```python
from build123d import *

# Parameters (mm, degrees)
BOSS_EXTRUDE2_DEPTH = 25
SKETCH4_R           = 4
CUT_EXTRUDE1_DEPTH  = 108.5257706
SKETCH6_R           = 4
CUT_EXTRUDE2_DEPTH  = 78.032036302
CUT_EXTRUDE3_DEPTH  = 78.032036302
SKETCH9_R           = 1.5
CUT_EXTRUDE4_DEPTH  = 78.032036302
SKETCH10_R          = 1.5
CUT_EXTRUDE5_DEPTH  = 108.5257706


with BuildPart() as part:
    # Sketch3 → Boss-Extrude2 (new body)
    with BuildSketch(Plane.XY):
        Polygon((-79.925523148, 45.386502584), (-27.042967192, 45.386502584), (-24.925523148, 45.386502584), (-24.925523148, -19.613497416), (-26.925523148, -19.613497416), (-26.925523148, 43.389953837), (-79.925523148, 43.389953837), (-79.925523148, -19.613497416), (-81.925523148, -19.613497416), (-81.925523148, 45.386502584), align=None)
    extrude(amount=BOSS_EXTRUDE2_DEPTH)

    # Sketch4 → Cut-Extrude1 (cut, through all)
    with BuildSketch(Plane(origin=(0, 45.386502584, 0), x_dir=(1, 0, 0), z_dir=(0, 1, 0))):
        with Locations(Location((-53.425523148, -12.5, 0), (0, 0, 270))):
            Circle(SKETCH4_R)
    extrude(amount=-CUT_EXTRUDE1_DEPTH, mode=Mode.SUBTRACT)

    # Sketch6 → Cut-Extrude2 (cut, through all)
    with BuildSketch(Plane.ZY.offset(81.925523148)):
        with Locations(Location((12.5, -5.613497416, 0), (0, 0, 270))):
            Circle(SKETCH6_R)
    extrude(amount=-CUT_EXTRUDE2_DEPTH, mode=Mode.SUBTRACT)

    # Sketch8 → Cut-Extrude3 (cut, through all)
    with BuildSketch(Plane.ZY.offset(81.925523148)):
        with BuildLine():
            Line((0, -19.613497416), (12.5, -19.613497416))
            ThreePointArc((12.5, -19.613497416), (3.661165213, -15.952332159), (0, -7.113497352))
            Line((0, -7.113497352), (0, -19.613497416))
        make_face()
        with BuildLine():
            Line((12.5, -19.613497416), (25, -19.613497416))
            Line((25, -19.613497416), (25, -7.113497416))
            ThreePointArc((25, -7.113497416), (21.338834765, -15.952332181), (12.5, -19.613497416))
        make_face()
    extrude(amount=-CUT_EXTRUDE3_DEPTH, mode=Mode.SUBTRACT)

    # Sketch9 → Cut-Extrude4 (cut, through all)
    with BuildSketch(Plane(origin=(-24.925523148, 0, 0), x_dir=(0, 0, -1), z_dir=(1, 0, 0))):
        with Locations(Location((-12.500004148, -12.613501564, 0), (0, 0, 90))):
            Circle(SKETCH9_R)
        with Locations(Location((-19.500008296, -5.613497416, 0), (0, 0, 90))):
            Circle(SKETCH9_R)
        with Locations(Location((-5.5, -5.613497416, 0), (0, 0, 90))):
            Circle(SKETCH9_R)
        with Locations(Location((-12.500004148, 1.386506731, 0), (0, 0, 90))):
            Circle(SKETCH9_R)
    extrude(amount=-CUT_EXTRUDE4_DEPTH, mode=Mode.SUBTRACT)

    # Sketch10 → Cut-Extrude5 (cut, through all)
    with BuildSketch(Plane(origin=(0, 45.386502584, 0), x_dir=(1, 0, 0), z_dir=(0, 1, 0))):
        with Locations(Location((-46.425523148, -12.499998866, 0), (0, 0, 270))):
            Circle(SKETCH10_R)
        with Locations(Location((-53.425523148, -5.499998866, 0), (0, 0, 270))):
            Circle(SKETCH10_R)
        with Locations(Location((-53.425523148, -19.499998866, 0), (0, 0, 270))):
            Circle(SKETCH10_R)
        with Locations(Location((-60.425523148, -12.499998866, 0), (0, 0, 270))):
            Circle(SKETCH10_R)
    extrude(amount=-CUT_EXTRUDE5_DEPTH, mode=Mode.SUBTRACT)


solid = part.part
```
Here's how the part is built. I have some questions about the finished solid (model axes, mm). A direction names the side the tool comes from. Coordinates: 2 decimals unless noted, no trailing zeros. Write each loop counter-clockwise with the first axis right and the second up, starting at its lowest first coordinate (ties: lowest second). Pieces come first, ordered by that corner, then holes. Notation, with made-up numbers: (47.5, -18) -> (61.5, -18) arc R28 ccw to (61.5, 20) -> close; hole circle Ø11 at (-16, 50.5). An arc over 180 degrees is marked (long way). Use a Markdown table: item, result. Add a question column.
(1) I'm going to push flat-ended pins straight in: P1, Ø2.5, axis at y = 1.39, z = 12.5, coming from the -X side; P2, Ø4, axis at x = -48, z = 11, coming from the -Y side. Where does each tip first touch, or does it pass through?
(2) Please list where these lines run through material, in increasing order: line 1 (X direction, y = 44.95, z = 12.5); line 2 (X direction, y = 11, z = 13.5); line 3 (Y direction, x = -30.5, z = 10.5).
(3) For faces 4 (the cylindrical face through (-51.94, 44.4, 5.3)), 5 (the flat face through (-26.926, 11, 12)), which set-ups out of +Z, -Z, +X, -X, +Y, -Y let a thin tool reach every point of the face, with its end or its side?
(4) If we section it at B-B, the plane z = 5.5: Write out the boundary of the cut face in (x, y).
(5) If we section it at D-D, the plane x = -36.5: Write out the boundary of the cut face in (y, z), and give its area (3 significant figures).
(6) If we section it at A-A, the plane y = 18.5: Write out the boundary of the cut face in (x, z), and give its area (3 significant figures).
(7) If we section it at C-C, the plane y = -5: State how many separate pieces and enclosed holes the cut face has, and give its area (3 significant figures).
(8) We'd pull the mould along X, two halves only. Please class faces 1 (the cylindrical face through (-80.9, -4.2, 6)), 2 (the flat face through (-53.05, 43.39, 17.88)), 3 (the flat face through (-24.926, 13, 12)): +X half, -X half, draft (parallel to the pull), parting line (faces both ways), or undercut.
Outcome:
| question | item | result |
|---|---|---|
| 1 | P1 | passes through |
| 1 | P2 | stops at y = 43.39 |
| 2 | line 1 | x = -81.93 to -61.93, -58.93 to -57.43, -49.43 to -47.93, -44.93 to -24.93 |
| 2 | line 2 | x = -81.93 to -79.93, -26.93 to -24.93 |
| 2 | line 3 | y = 43.39 to 45.39 |
| 3 | face 4 | +Y, -Y |
| 3 | face 5 | +Z, -Z, -Y |
| 4 | outline | (-81.93, -17.47) -> (-79.93, -17.47) -> (-79.93, -7.11) -> (-81.93, -7.11) -> close; (-81.93, -4.11) -> (-79.93, -4.11) -> (-79.93, 43.39) -> (-54.93, 43.39) -> (-54.93, 45.39) -> (-81.93, 45.39) -> close; (-51.93, 43.39) -> (-26.93, 43.39) -> (-26.93, -4.11) -> (-24.93, -4.11) -> (-24.93, 45.39) -> (-51.93, 45.39) -> close; (-26.93, -17.47) -> (-24.93, -17.47) -> (-24.93, -7.11) -> (-26.93, -7.11) -> close |
| 5 | outline | (43.39, 0) -> (45.39, 0) -> (45.39, 25) -> (43.39, 25) -> close |
| 5 | area | 49.9 mm^2 |
| 6 | outline | (-81.93, 0) -> (-79.93, 0) -> (-79.93, 25) -> (-81.93, 25) -> close; (-26.93, 0) -> (-24.93, 0) -> (-24.93, 25) -> (-26.93, 25) -> close |
| 6 | area | 100 mm^2 |
| 7 | separate pieces | 8 |
| 7 | enclosed holes | 0 |
| 7 | area | 46.5 mm^2 |
| 8 | face 1 | draft |
| 8 | face 2 | undercut |
| 8 | face 3 | +X half |
